from build123d import *

# Parameters (mm, degrees)
SKETCH1_W           = 95
SKETCH1_H           = 260
BOSS_EXTRUDE1_DEPTH = 12
SKETCH3_R           = 3.5
CUT_EXTRUDE1_DEPTH  = 13
SKETCH4_R           = 1.55
CUT_EXTRUDE2_DEPTH  = 13


with BuildPart() as part:
    # Sketch1 → Boss-Extrude1 (new body)
    with BuildSketch(Plane.XY):
        Rectangle(SKETCH1_W, SKETCH1_H)
    extrude(amount=BOSS_EXTRUDE1_DEPTH)

    # Sketch3 → Cut-Extrude1 (cut, through all)
    with BuildSketch(Plane.XY.offset(12)):
        with Locations((-27.5, -110)):
            Circle(SKETCH3_R)
        with Locations((27.5, -110)):
            Circle(SKETCH3_R)
    extrude(amount=-CUT_EXTRUDE1_DEPTH, mode=Mode.SUBTRACT)

    # Sketch4 → Cut-Extrude2 (cut, through all)
    with BuildSketch(Plane.XY.offset(12)):
        with Locations((-30, -90)):
            Circle(SKETCH4_R)
        with Locations((30, -90)):
            Circle(SKETCH4_R)
        with Locations((30, 124)):
            Circle(SKETCH4_R)
        with Locations((-30, 124)):
            Circle(SKETCH4_R)
    extrude(amount=-CUT_EXTRUDE2_DEPTH, mode=Mode.SUBTRACT)


solid = part.part
Source: CAD feature listing. Evaluate the final solid. Frame: model axes, mm. Coordinates: 2 decimals unless noted, no trailing zeros. Loops run counter-clockwise (first coordinate to the right, second up) from the corner with the lowest first, then second, coordinate; pieces in that order, holes last. Notation, with made-up numbers: M -7,76 L 15,76 A22 cw 15,100 Z; hole C 68,42.25 d10. An arc over 180 degrees is marked long. Answer in a Markdown table with one row per item.
Q1. Ray query, probe 1 along X at (y, z) = (-90, 4); probe 2 along Y at (x, z) = (-27, 1.5); probe 3 along Y at (x, z) = (30, 7.5). Return the intervals inside material, ascending. Write a range as from..to.
Answers below:
| item | result |
|---|---|
| probe 1 | x = -47.5..-31.55, -28.45..28.45, 31.55..47.5 |
| probe 2 | y = -130..-113.46, -106.54..130 |
| probe 3 | y = -130..-112.45, -107.55..-91.55, -88.45..122.45, 125.55..130 |
Q2. Draft query along Y for faces 1 (the flat face through (-1, -130, 6)), 2 (the cylindrical face through (-28.259, -113.417, 6.084)), 3 (the flat face through (-1, 2, 12)), 4 (the cylindrical face through (26.741, -113.417, 6.084)). Return one class per face: pulls with the +Y half, pulls with the -Y half, needs draft (parallel to the pull), parting line crosses it, or undercut.
Answers below:
| item | result |
|---|---|
| face 1 | pulls with the -Y half |
| face 2 | undercut |
| face 3 | needs draft |
| face 4 | undercut |
Q3. Section A-A on y = -110. Return the cut outline in (x, z), plus the area to 3 significant figures.
Answers below:
| item | result |
|---|---|
| outline | M -47.5,0 L -31,0 L -31,12 L -47.5,12 Z; M -24,0 L 24,0 L 24,12 L -24,12 Z; M 31,0 L 47.5,0 L 47.5,12 L 31,12 Z |
| area | 972 mm^2 |
